from build123d import *

# Parameters (mm, degrees)
BOSS_EXTRUDE1_DEPTH = 5
SKETCH2_R           = 2.25
CUT_EXTRUDE1_DEPTH  = 44.703546767


with BuildPart() as part:
    # Sketch1 → Boss-Extrude1 (new, symmetric)
    with BuildSketch(Plane.XY):
        with BuildLine():
            Line((-17, 0), (17, 0))
            ThreePointArc((17, 0), (17.707106781, 0.292893219), (18, 1))
            Line((18, 1), (18, 18))
            ThreePointArc((18, 18), (19.757359313, 22.242640687), (24, 24))
            Line((24, 24), (34, 24))
            Line((34, 24), (34, 21))
            Line((34, 21), (24, 21))
            ThreePointArc((24, 21), (21.878679656, 20.121320344), (21, 18))
            Line((21, 18), (21, 1))
            ThreePointArc((21, 1), (19.828427125, -1.828427125), (17, -3))
            Line((17, -3), (-17, -3))
            ThreePointArc((-17, -3), (-19.828427125, -1.828427125), (-21, 1))
            Line((-21, 1), (-21, 18))
            ThreePointArc((-21, 18), (-21.878679656, 20.121320344), (-24, 21))
            Line((-24, 21), (-34, 21))
            Line((-34, 21), (-34, 24))
            Line((-34, 24), (-24, 24))
            ThreePointArc((-24, 24), (-19.757359313, 22.242640687), (-18, 18))
            Line((-18, 18), (-18, 1))
            ThreePointArc((-18, 1), (-17.707106781, 0.292893219), (-17, 0))
        make_face()
    extrude(amount=BOSS_EXTRUDE1_DEPTH, both=True)

    # Sketch2 → Cut-Extrude1 (cut, through all)
    with BuildSketch(Plane(origin=(0, 24, 0), x_dir=(1, 0, 0), z_dir=(0, 1, 0))):
        with Locations(Location((-29, 0, 0), (0, 0, 180))):
            Circle(SKETCH2_R)
    cut_extrude1 = extrude(amount=-CUT_EXTRUDE1_DEPTH, mode=Mode.SUBTRACT)

    # Mirror1: Cut-Extrude1 across plane
    add(cut_extrude1.mirror(Plane(origin=(0, 0, 0), x_dir=(0, 0, 1), z_dir=(1, 0, 0))), mode=Mode.SUBTRACT)


solid = part.part
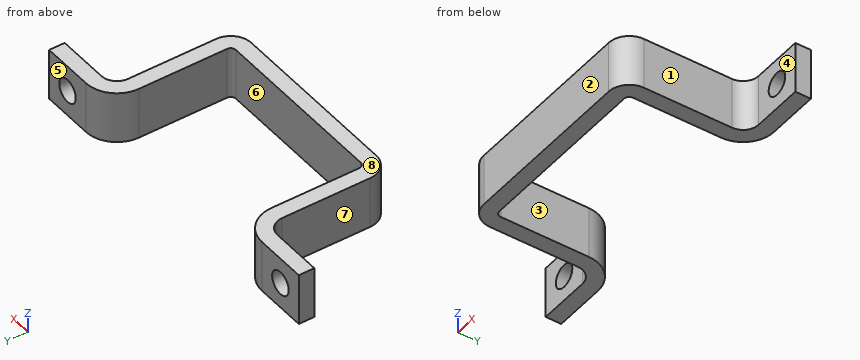
Verification items for the finished model (mm, model axes). Face numbers are marked on the shaded views. A direction names the side the tool comes from. Round coordinates to 2 decimals unless told otherwise and drop trailing zeros. Loops run counter-clockwise (first coordinate to the right, second up) from the corner with the lowest first, then second, coordinate; pieces in that order, holes last. Notation, with made-up numbers: (55, 43) - (91, 43) arc R33 cw to (91, 81) - close; hole circle Ø11 at (-12, 6). An arc over 180 degrees is marked (long way). Use a Markdown table: item, result. Add a question column.
1. Release check for a two-part mould opening along X. For the marked faces 1, 2 and 3 record: released by +X, released by -X, zero draft, split by the parting line, or undercut.
2. Section check A-A, the plane x = -29. Record the boundary of the cut face in (y, z).
3. Section check B-B, the plane z = 0. Record the boundary of the cut face in (x, y).
4. Access from +Z, -Z, +X, -X, +Y, -Y to the whole of each face (thin tool, end or side, straight path). Record for the marked faces 4, 5, 6, 7 and 8.
5. Thickness scan on probe 1 along X at (y, z) = (5, 3.25); probe 2 along Z at (x, y) = (-29, 22.3); probe 3 along Y at (x, z) = (24.5, 0). Record the ranges inside material, lowest first. Write a range as [from, to].
6. Gauge pin test, flat ends, axial feed: pin 1 (3 mm diameter, centred on y = 9.5, z = 0.5, fed in from +X); pin 2 (3 mm diameter, centred on y = 18, z = 0.5, fed in from +X); pin 3 (3.5 mm diameter, centred on x = -29, z = 0, fed in from -Y); pin 4 (4 mm diameter, centred on y = 16.5, z = -3.5, fed in from -X). Record the tip position at first contact, or that the pin passes through.
7. Section check D-D, the plane z = -3.25. Record the boundary of the cut face in (x, y).
8. Section check C-C, the plane y = 4. Record the boundary of the cut face in (x, z), plus the area to 3 significant figures.
Checks:
| question | item | result |
|---|---|---|
| 1 | face 1 | released by +X |
| 1 | face 2 | zero draft |
| 1 | face 3 | undercut |
| 2 | outline | (21, -5) - (24, -5) - (24, -2.25) - (21, -2.25) - close; (21, 2.25) - (24, 2.25) - (24, 5) - (21, 5) - close |
| 3 | outline | (-34, 21) - (-31.25, 21) - (-31.25, 24) - (-34, 24) - close; (-26.75, 21) - (-24, 21) arc R3 cw to (-21, 18) - (-21, 1) arc R4 ccw to (-17, -3) - (17, -3) arc R4 ccw to (21, 1) - (21, 18) arc R3 cw to (24, 21) - (26.75, 21) - (26.75, 24) - (24, 24) arc R6 ccw to (18, 18) - (18, 1) arc R1 cw to (17, 0) - (-17, 0) arc R1 cw to (-18, 1) - (-18, 18) arc R6 ccw to (-24, 24) - (-26.75, 24) - close; (31.25, 21) - (34, 21) - (34, 24) - (31.25, 24) - close |
| 4 | face 4 | +Z, -Z, +X, -Y |
| 4 | face 5 | +Z, -Z, +X, -X, +Y |
| 4 | face 6 | +Z, -Z, +Y |
| 4 | face 7 | +Z, -Z, -X, -Y |
| 4 | face 8 | +Z, +X, -X, +Y, -Y |
| 5 | probe 1 | x = [-21, -18], [18, 21] |
| 5 | probe 2 | z = [-5, -2.25], [2.25, 5] |
| 5 | probe 3 | y = [21, 24] |
| 6 | pin 1 | stops at x = 21 |
| 6 | pin 2 | stops at x = 21.4 |
| 6 | pin 3 | passes through |
| 6 | pin 4 | stops at x = -21.04 |
| 7 | outline | (-34, 21) - (-24, 21) arc R3 cw to (-21, 18) - (-21, 1) arc R4 ccw to (-17, -3) - (17, -3) arc R4 ccw to (21, 1) - (21, 18) arc R3 cw to (24, 21) - (34, 21) - (34, 24) - (24, 24) arc R6 ccw to (18, 18) - (18, 1) arc R1 cw to (17, 0) - (-17, 0) arc R1 cw to (-18, 1) - (-18, 18) arc R6 ccw to (-24, 24) - (-34, 24) - close |
| 8 | outline | (-21, -5) - (-18, -5) - (-18, 5) - (-21, 5) - close; (18, -5) - (21, -5) - (21, 5) - (18, 5) - close |
| 8 | area | 60.0 mm^2 |
